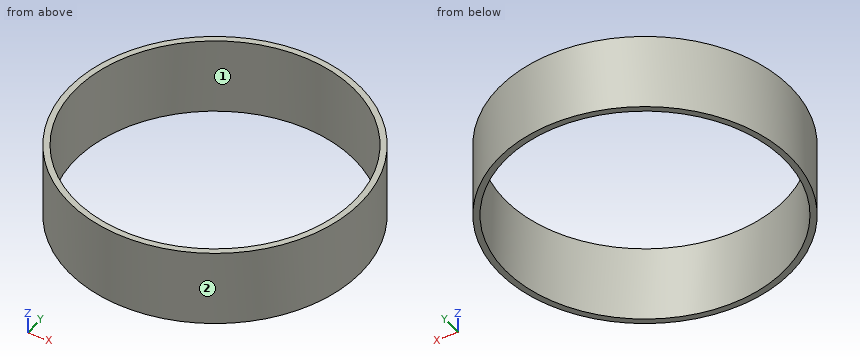
from build123d import *

# Parameters (mm, degrees)
CYLINDER008_R     = 73.025
CYLINDER008_DEPTH = 40
CYLINDER002_R     = 76.2
CYLINDER002_DEPTH = 40


with BuildPart() as chamberwall001:
    # Cylinder008 → Cylinder008 (new body)
    with BuildSketch(Plane(origin=(105, 148, 0), x_dir=(1, 0, 0), z_dir=(0, 0, 1))):
        Circle(CYLINDER008_R)
    extrude(amount=CYLINDER008_DEPTH)


with BuildPart() as chamberwall002:
    # Cylinder002 → Cylinder002 (new body)
    with BuildSketch(Plane(origin=(105, 148, 0), x_dir=(1, 0, 0), z_dir=(0, 0, 1))):
        Circle(CYLINDER002_R)
    extrude(amount=CYLINDER002_DEPTH)

    # Cut: cut ChamberWall001
    add(chamberwall001.part, mode=Mode.SUBTRACT)


with BuildPart() as chamberwall002_1:
    # Cut placement: moved
    add(chamberwall002.part.moved(Location((0, 0, 19))))


solid = chamberwall002_1.part
Verification items for the finished model (mm, model axes). Face numbers are marked on the shaded views. Give positions to 0.01 mm unless a question says otherwise; leave off trailing zeros. Write each loop counter-clockwise with the first axis right and the second up, starting at its lowest first coordinate (ties: lowest second). Pieces come first, ordered by that corner, then holes.
(1) Cross-section at B-B (x = 105). Enter the section's corners in (y, z) (3 decimals), plus the area to 3 significant figures.
(2) Cross-section at A-A (y = 148). Enter the section's corners in (x, z) (3 decimals).
(3) Mould release check, pull along X, two halves, no side actions. Record for the marked faces 1 and 2: +X half, -X half, draft (parallel to the pull), parting line (faces both ways), or undercut.
(4) Material ranges on line 1 (Y direction, x = 105, z = 33.5) (3 decimals); line 2 (Y direction, x = 100, z = 31); line 3 (X direction, y = 127, z = 29.5), recorded low to high.
(5) Cross-section at C-C (z = 44.5). Enter the section's corners in (x, y) (3 decimals).
(6) Gauge pin test, flat ends, axial feed: pin 1 (6 mm diameter, centred on x = 111, z = 52, fed in from +Y); pin 2 (8 mm diameter, centred on y = 157.5, z = 52.5, fed in from +X); pin 3 (5 mm diameter, centred on y = 119.5, z = 46, fed in from +X). Record the tip position at first contact, or that the pin passes through.
Worked out:
1. outline: (71.8, 19) - (74.975, 19) - (74.975, 59) - (71.8, 59) - close; (221.025, 19) - (224.2, 19) - (224.2, 59) - (221.025, 59) - close
1. area: 254 mm2
2. outline: (28.8, 19) - (31.975, 19) - (31.975, 59) - (28.8, 59) - close; (178.025, 19) - (181.2, 19) - (181.2, 59) - (178.025, 59) - close
3. face 1: undercut
3. face 2: parting line
4. line 1: y = 71.8 to 74.975, 221.025 to 224.2
4. line 2: y = 71.96 to 75.15, 220.85 to 224.04
4. line 3: x = 31.75 to 35.06, 174.94 to 178.25
5. outline: circle Ø152.4 at (105, 148); hole circle Ø146.05 at (105, 148)
6. pin 1: stops at y = 224.14
6. pin 2: stops at x = 181
6. pin 3: stops at x = 176.63
